Work out the finished part from the listing and answer in its coordinate system (mm). A direction names the side the tool comes from. Coordinates: 2 decimals unless noted, no trailing zeros. Loops run counter-clockwise (first coordinate to the right, second up) from the corner with the lowest first, then second, coordinate; pieces in that order, holes last. Notation, with made-up numbers: (34, 62) - (79, 62) arc R16 ccw to (79, 69) - close; hole circle Ø10 at (67, 84.5). An arc over 180 degrees is marked (long way). Write each question's results on one line, items separated by ' | '. Start each with the question number.
Item 1: Each of these flat-tipped pins is pushed along its axis until it touches: pin 1 Ø1 at (y, z) = (-12.5, -59.5) entering from -X; pin 2 Ø7 at (y, z) = (0, -79.5) entering from -X; pin 3 Ø4 at (x, z) = (-38.1, -38.1) entering from -Y (3 decimals). Where does it stop, or does it pass through?
Item 2: Section D-D, the plane y = 8 is taken. Write down the section's boundary in (x, z) (3 decimals).
Item 3: For a pull along Y with two mould halves and no side action, classify faces 1 (the face through (-32, 0, -76.2)), 2 (the face through (-61.89, 17.485, -38.678)), 3 (the face through (-31.784, 16.152, -38.239)) as +Y half, -Y half, draft (parallel to the pull), parting line (faces both ways), or undercut.
Item 4: Section B-B, the plane z = -38.1 is taken. Count the separate pieces of the cut face and the enclosed holes in it, plus the area to 3 significant figures.
Item 5: A tool of negligible diameter and unlimited length cuts with its end or side. For faces 4 (the face through (-38.4, -13.335, -46)), 5 (the face through (-38.1, -16, -51)), 6 (the face through (-55, -5.08, -79)), from which of +Z, -Z, +X, -X, +Y, -Y can it reach the whole face along a straight path? Write none if from no direction.
Item 6: Section C-C, the plane z = -6.5 is taken. Write down the section's boundary in (x, y) (3 decimals), plus the area to 3 significant figures.
Item 7: Consider probe 1 along X at (y, z) = (15, -38); probe 2 along Z at (x, y) = (-26.5, 7); probe 3 along Y at (x, z) = (-1.5, -61.5) (3 decimals). Determine where each line is inside the solid, lowest interval first. Write a range as [from, to].
Item 8: Section A-A, the plane x = -16 is taken. Write down the section's boundary in (y, z) (3 decimals), plus the area to 3 significant figures.
Autodesk Inventor part; units mm, degrees
ref_plane "YZ Plane" through (0, 0, 0) normal (1, 0, 0) x (0, 1, 0)
ref_plane "XZ Plane" through (0, 0, 0) normal (0, 1, 0) x (-1, 0, 0)
ref_plane "XY Plane" through (0, 0, 0) normal (0, 0, 1) x (1, 0, 0)
sketch "Sketch1" plane through (0, 0, 0) normal (0, 1, 0) x (-1, 0, 0)
  line L0 (0, 0) -> (76.2, 0)
  line L1 (76.2, 0) -> (76.2, -76.2)
  line L2 (76.2, -76.2) -> (0, -76.2)
  line L3 (0, -76.2) -> (0, 0)
  line L4 (-6.35, 6.35) -> (76.2, 6.35)
  line L5 (76.2, -82.55) -> (-6.35, -82.55)
  line L6 (-6.35, -82.55) -> (-6.35, 6.35)
  line L7 (76.2, 6.35) -> (63.5, 6.35)
  line L8 (63.5, 6.35) -> (63.5, -82.55)
  line L9 (76.2, -38.1) -> (0, -38.1)
  line L10 (38.1, 0) -> (38.1, -76.2)
  circle A0 centre (38.1, -38.1) radius 3.048
  circle A1 centre (38.1, -38.1) radius 1.5875
  circle A2 centre (38.1, -38.1) radius 6.3171
  circle A3 centre (38.1, -38.1) radius 19.2182
  point P0 (63.5, 0)
  point P1 (63.5, -76.2)
  point P2 (38.1, -57.3182)
  point P3 (38.1, -44.4171)
  point P4 (38.1, -31.7829)
  point P5 (38.1, -18.8818)
  dimension "d0" = 76.2
  dimension "d1" = 76.2
  dimension "d2" = 6.35
  dimension "d3" = 6.35
  dimension "d4" = 6.35
  dimension "d6" = 12.7
  dimension "d7" = 6.096
  dimension "d12" = 3.175
extrude "Extrusion1" add sketch "Sketch1" along normal mid plane 38.1 contours L3 L2 L8 L5 L6 L4 L0 | L0 L10 A3 L9 L3 | L0 L8 L9 A3 L10 | L9 A3 L10 L2 L3 | A3 L9 A2 L10 | L10 A2 L9 A3 | L9 A2 L10 A3 | L8 L2 L10 A3 L9 | A2 L9 A0 L10 | L10 A0 L9 A2 | A3 L10 A2 L9 | L9 A0 L10 A2 | A0 L9 A1 L10 | L10 A1 L9 A0 | A2 L10 A0 L9 | L9 A1 L10 A0 | A1 L9 L10 | L10 L9 A1 | A0 L10 A1 L9 | L9 L10 A1 | L9 A1 L10
extrude "Extrusion2" cut sketch "Sketch1" along normal mid plane 26.67 contours L0 L10 A3 L9 L3 | L0 L8 L9 A3 L10 | L9 A3 L10 L2 L3 | A3 L9 A2 L10 | L10 A2 L9 A3 | L9 A2 L10 A3 | L8 L2 L10 A3 L9 | A2 L9 A0 L10 | L10 A0 L9 A2 | A3 L10 A2 L9 | L9 A0 L10 A2 | A0 L9 A1 L10 | L10 A1 L9 A0 | A2 L10 A0 L9 | L9 A1 L10 A0 | A1 L9 L10 | L10 L9 A1 | A0 L10 A1 L9 | L9 L10 A1 | L9 A1 L10
extrude "Extrusion3" cut sketch "Sketch1" along normal blind 26.67 contours A1 L9 L10 | L10 L9 A1 | L9 L10 A1 | L9 A1 L10
extrude "Extrusion4" cut sketch "Sketch1" against normal blind 26.67 contours A0 L9 A1 L10 | L10 A1 L9 A0 | L9 A1 L10 A0 | A1 L9 L10 | L10 L9 A1 | A0 L10 A1 L9 | L9 L10 A1 | L9 A1 L10
extrude "Extrusion5" cut sketch "Sketch1" along normal mid plane 76.2 contours L10 A2 L9 A3 | L9 A2 L10 A3 picked at (24.03, -33.4265) picked at (23.3428, -39.5255)
chamfer "Chamfer1" distance 3.175 angle 45 12 edges at (6.35, -19.05, -38.1) (6.35, 0, -82.55) (6.35, 19.05, -38.1) (6.35, 0, 6.35) (-28.575, -19.05, 6.35) (-28.575, -19.05, -82.55) (-28.575, 19.05, 6.35) (-28.575, 19.05, -82.55) (-63.5, 0, -82.55) (-63.5, 19.05, -38.1) (-63.5, 0, 6.35) (-63.5, -19.05, -38.1)
sketch "Sketch2" plane through (-60.325, 15.875, 6.35) normal (0, 0, 1) x (1, 0, 0)
  line L0 (60.325, -15.875) -> (-14.3464, -15.875)
  line L1 (-14.3464, -15.875) -> (-14.3464, -10.795)
  line L2 (-3.175, -31.75) -> (-3.175, 0)
  line L3 (-14.3464, -10.795) -> (60.325, -10.795)
  line L4 (60.325, -29.21) -> (60.325, -2.54)
  line L5 (60.325, -10.795) -> (60.325, -20.955)
  line L6 (60.325, -20.955) -> (-14.3464, -20.955)
  line L7 (-14.3464, -20.955) -> (-14.3464, -15.875)
  line L8 (12.9951, -20.955) -> (12.9951, -10.795)
  line L9 (35.8551, -10.795) -> (35.8551, -20.955)
  dimension "d22" = 5.08
  dimension "d23" = 10.16
  dimension "d26" = 24.4699
  dimension "d27" = 22.86
extrude "Extrusion6" cut sketch "Sketch2" against normal blind 127 contours L4 L6 L9 L0 | L0 L9 L3 L4 | L8 L6 L2 L0 | L0 L2 L3 L8 | L2 L6 L7 L0 | L0 L1 L3 L2
sketch "Sketch3" plane through (-60.325, -15.875, 6.35) normal (0, 0, 1) x (1, 0, 0)
  point P0 (60.325, 15.875)
properties part number "Flywheel Cutting Jig"
Answer key:
1) pin 1: stops at x = 0 | pin 2: stops at x = -47.33 | pin 3: stops at y = 13.335
2) outline: (-63.5, -79.375) - (-60.325, -82.55) - (3.175, -82.55) - (6.35, -79.375) - (6.35, 3.175) - (3.175, 6.35) - (-60.325, 6.35) - (-63.5, 3.175) - (-63.5, 0) - (0, 0) - (0, -76.2) - (-63.5, -76.2) - close
3) face 1: undercut | face 2: +Y half | face 3: draft
4) separate pieces: 5 | enclosed holes: 0 | area: 747 mm^2
5) face 4: -X | face 5: +Y, -Y | face 6: +Z, -Z, -X
6) outline: (-63.5, -15.875) - (-60.325, -19.05) - (3.175, -19.05) - (6.35, -15.875) - (6.35, 15.875) - (3.175, 19.05) - (-60.325, 19.05) - (-63.5, 15.875) - (-63.5, 13.335) - (0, 13.335) - (0, -13.335) - (-63.5, -13.335) - close | area: 948 mm^2
7) probe 1: x = [-63.5, -39.68], [-36.52, -31.78], [-18.88, 6.35] | probe 2: z = [-82.55, -76.2], [0, 6.35] | probe 3: y = [-19.05, -13.335], [13.335, 19.05]
8) outline: (-19.05, -79.375) - (-15.875, -82.55) - (-5.08, -82.55) - (-5.08, -76.2) - (-13.335, -76.2) - (-13.335, 0) - (-5.08, 0) - (-5.08, 6.35) - (-15.875, 6.35) - (-19.05, 3.175) - close; (5.08, -82.55) - (15.875, -82.55) - (19.05, -79.375) - (19.05, 3.175) - (15.875, 6.35) - (5.08, 6.35) - (5.08, 0) - (13.335, 0) - (13.335, -76.2) - (5.08, -76.2) - close | area: 1,210 mm^2
